Model file for the job. Use its own axes, mm. A direction names the side the tool comes from. Give positions to 0.01 mm unless a question says otherwise; leave off trailing zeros. Loops run counter-clockwise (first coordinate to the right, second up) from the corner with the lowest first, then second, coordinate; pieces in that order, holes last. Notation, with made-up numbers: M 45,58.5 L 87,58.5 A34 cw 87,97.5 Z; hole C 52,34 d3. An arc over 180 degrees is marked long. Answer in a Markdown table with one row per item.
```python
from build123d import *

# Parameters (mm, degrees)
F0_W          = 38.1
F0_H          = 38.1
F0_W_2        = 33.02
F0_H_2        = 33.02
F0_W_3        = 25.4
F0_H_3        = 25.4
F1_DEPTH      = 4.445
F1_DEPTH_BACK = 4.445
F2_DEPTH      = 3.175
F2_DEPTH_BACK = 3.175
F3_R          = 2.54
F4_R          = 2.54
F5_R          = 5.08


with BuildPart() as f1:
    # F0 (on Top) → F1 (new body, two sides)
    with BuildSketch(Plane.XY) as f1_sk:
        Rectangle(F0_W, F0_H)
        Rectangle(F0_W_2, F0_H_2, mode=Mode.SUBTRACT)
        Rectangle(F0_W_2, F0_H_2)
        Rectangle(F0_W_3, F0_H_3, mode=Mode.SUBTRACT)
    extrude(amount=F1_DEPTH)
    extrude(f1_sk.sketch, amount=-F1_DEPTH_BACK)

    # F0 (on Top) → F2 (cut, two sides)
    with BuildSketch(Plane.XY) as f2_sk:
        Rectangle(F0_W_2, F0_H_2)
        Rectangle(F0_W_3, F0_H_3, mode=Mode.SUBTRACT)
    extrude(amount=F2_DEPTH, mode=Mode.SUBTRACT)
    extrude(f2_sk.sketch, amount=-F2_DEPTH_BACK, mode=Mode.SUBTRACT)

    # F3
    f3_edges = [f1.edges().sort_by_distance(p)[0] for p in [
        (-16.51, 0, -3.175),
        (0, 16.51, -3.175),
        (16.51, 0, -3.175),
        (0, -16.51, -3.175),
    ]]
    fillet(f3_edges, radius=F3_R)

    # F4
    f4_edges = [f1.edges().sort_by_distance(p)[0] for p in [
        (0, 16.51, 3.175),
        (16.51, 0, 3.175),
        (0, -16.51, 3.175),
        (-16.51, 0, 3.175),
    ]]
    fillet(f4_edges, radius=F4_R)

    # F5
    f5_edges = [f1.edges().sort_by_distance(p)[0] for p in [
        (19.05, 0, 4.445),
        (0, 19.05, 4.445),
        (-19.05, 0, 4.445),
        (0, -19.05, 4.445),
    ]]
    fillet(f5_edges, radius=F5_R)


solid = f1.part
```
(1) Saw through at B-B, the plane z = -4. Give the cut face in (x, y).
Established:
| item | result |
|---|---|
| outline | M -19.05,-19.05 L 19.05,-19.05 L 19.05,19.05 L -19.05,19.05 Z; hole M -12.7,-12.7 L 12.7,-12.7 L 12.7,12.7 L -12.7,12.7 Z |
(2) Wall check: L1, parallel to X at y = 2, z = -3.5; L2, parallel to X at y = -14, z = -0.5. Give the ranges that are in metal, low to high.
Established:
| item | result |
|---|---|
| L1 | x = -19.05 to -12.7, 12.7 to 19.05 |
| L2 | x = -19.05 to -16.51, 16.51 to 19.05 |
(3) Saw through at D-D, the plane z = 2. Give the cut face in (x, y), and give its area (3 significant figures).
Established:
| item | result |
|---|---|
| outline | M -18.31,-18.31 L 18.31,-18.31 L 18.31,18.31 L -18.31,18.31 Z; hole M -16.11,-16.11 L 16.11,-16.11 L 16.11,16.11 L -16.11,16.11 Z |
| area | 303 mm2 |
(4) Saw through at A-A, the plane y = -11.5. Give the cut face in (x, z) (3 decimals).
Established:
| item | result |
|---|---|
| outline | M -19.05,-4.445 L -12.7,-4.445 L -12.7,-3.175 L -13.97,-3.175 A2.54 cw -16.51,-0.635 L -16.51,0.635 A2.54 cw -13.97,3.175 L -12.7,3.175 L -12.7,4.445 L -13.97,4.445 A5.08 ccw -19.05,-0.635 Z; M 12.7,-4.445 L 19.05,-4.445 L 19.05,-0.635 A5.08 ccw 13.97,4.445 L 12.7,4.445 L 12.7,3.175 L 13.97,3.175 A2.54 cw 16.51,0.635 L 16.51,-0.635 A2.54 cw 13.97,-3.175 L 12.7,-3.175 Z |
(5) Which spindle directions (+Z, -Z, +X, -X, +Y, -Y) get a long thin tool onto all of the face, cutting with end or side? Do faces 1 (the flat face through (12.7, 0, -4)), 2 (the cylindrical face through (-15.746, 0.231, -2.451)), 3 (the cylindrical face through (0.27, 17.52, 3)). Say none if no direction does.
Established:
| item | result |
|---|---|
| face 1 | +Z, -Z |
| face 2 | none |
| face 3 | +Z, +X, -X, +Y |
(6) Flat gauge pins, fed straight in: P1, Ø1.4, axis at y = 5.5, z = 0, coming from the -X side; P2, Ø0.6, axis at x = -5, z = 4, coming from the +Y side; P3, Ø2, axis at y = 4.5, z = 1.5, coming from the +X side; P4, Ø0.6, axis at x = 4, z = 3.5, coming from the -Y side. Where does each tip first touch, or does it go through?
Established:
| item | result |
|---|---|
| P1 | stops at x = -19.05 |
| P2 | stops at y = 16.62 |
| P3 | stops at x = 18.92 |
| P4 | stops at y = -17.3 |
(7) Mould opens along X. For faces 4 (the cylindrical face through (0.27, -17.52, 3)), 5 (the cylindrical face through (-17.52, 0.27, 3)), 6 (the cylindrical face through (0.231, 15.786, 2.411)), 7 (the flat face through (19.05, 0, -3)) say: pulls with the +X half, pulls with the -X half, needs draft (parallel to the pull), parting line crosses it, or undercut.
Established:
| item | result |
|---|---|
| face 4 | needs draft |
| face 5 | pulls with the -X half |
| face 6 | undercut |
| face 7 | pulls with the +X half |
